Verification items for the finished model (mm, model axes). A direction names the side the tool comes from. Round coordinates to 2 decimals unless told otherwise and drop trailing zeros. Loops run counter-clockwise (first coordinate to the right, second up) from the corner with the lowest first, then second, coordinate; pieces in that order, holes last. Notation, with made-up numbers: M -24.75,10.25 L 33.25,10.25 A24 cw 33.25,37.25 Z; hole C 8,-25 d1. An arc over 180 degrees is marked long. One line per item, written item: value.
Autodesk Inventor part; units mm, degrees
ref_plane "YZ Plane" through (0, 0, 0) normal (1, 0, 0) x (0, 1, 0)
ref_plane "XZ Plane" through (0, 0, 0) normal (0, 1, 0) x (-1, 0, 0)
ref_plane "XY Plane" through (0, 0, 0) normal (0, 0, 1) x (1, 0, 0)
sketch "Sketch1" plane through (0, 0, 0) normal (0, 0, 1) x (1, 0, 0)
  circle A0 centre (0, 0) radius 38.1
  circle A1 centre (0, 0) radius 19.05
  dimension "d0" = 76.2
  dimension "d1" = 38.1
extrude "Extrusion1" add sketch "Sketch1" along normal blind 5.08
sketch "Sketch2" plane through (0, 0, 0) normal (0, 0, -1) x (-1, 0, 0)
  circle A0 centre (0, 0) radius 46.5667
  circle A1 centre (0, 0) radius 38.1
  dimension "d8" = 8.4667
extrude "Extrusion2" add sketch "Sketch2" against normal blind 20.2142
sketch "Sketch3" plane through (0, 0, 20.2142) normal (0, 0, 1) x (1, 0, 0)
  circle A0 centre (0, 0) radius 46.5667 construction
  arc A1 (23.2833, 40.3279) -> (0, 46.5667) centre (0, 0) ccw
  line L0 (0, 0) -> (23.2833, 40.3279) construction
  line L1 (0, 0) -> (0, 46.5667) construction
  circle A2 centre (0, 0) radius 38.1
  circle A3 centre (0, 0) radius 46.5667
  circle A4 centre (0, 0) radius 38.1
  line L2 (0, 38.1) -> (0, 46.5667)
  line L3 (19.05, 32.9956) -> (23.2833, 40.3279)
  arc A5 (19.05, 32.9956) -> (0, 38.1) centre (0, 0) ccw
  dimension "d9" = 30
extrude "Extrusion3" cut sketch "Sketch3" against normal blind 8.4667 contours L3 A2 L2 A1
pattern_circular "Circular Pattern1" count 6 over 360 about axis through (0, 0, 0) along (0, 0, 1) of "Extrusion3"
sketch "Sketch4" plane through (0, 0, 20.2142) normal (0, 0, 1) x (1, 0, 0)
  line L0 (-40.8909, 10.9567) -> (-10.9567, 40.8909)
  line L1 (-10.9567, 40.8909) -> (29.9342, 29.9342)
  line L2 (29.9342, 29.9342) -> (40.8909, -10.9567)
  line L3 (40.8909, -10.9567) -> (10.9567, -40.8909)
  line L4 (10.9567, -40.8909) -> (-29.9342, -29.9342)
  line L5 (-29.9342, -29.9342) -> (-40.8909, 10.9567)
  line L6 (-23.2833, 40.3279) -> (-19.05, 32.9956)
  arc A0 (0, 38.1) -> (-19.05, 32.9956) centre (0, 0) ccw
  line L7 (0, 38.1) -> (0, 46.5667)
  arc A1 (0, 46.5667) -> (-23.2833, 40.3279) centre (0, 0) ccw
  arc A2 (0, 38.1) -> (-19.05, 32.9956) centre (0, 0) ccw
  line L8 (-9.861, 36.8018) -> (-12.0523, 44.9799)
  arc A3 (0, 46.5667) -> (-23.2833, 40.3279) centre (0, 0) ccw
hole "Hole1" at (-10.9567, 40.8909, 20.2142) at (29.9342, 29.9342, 20.2142) at (-40.8909, 10.9567, 20.2142) at (-29.9342, -29.9342, 20.2142) at (10.9567, -40.8909, 20.2142) at (40.8909, -10.9567, 20.2142) direction (0, 0, -1) diameter 6 end through all
properties part number "Stator"
(1) Tool access check on faces 1 (the face through (0, -42, 16)), 2 (the face through (0, 42, 16)), 3 (the face through (40, 10, 11.748)). Record the directions out of +Z, -Z, +X, -X, +Y, -Y that give a thin tool (end or side, any length) a straight path to the whole face; none if there is none.
Completed:
face 1: +Z, -Y
face 2: +Z, +Y
face 3: +Z, +X
(2) Sectioned sample at D-D on z = 2.75. Enter the section's corners in (x, y), and give its area (3 significant figures).
Completed:
outline: C 0,0 d93.13; hole C -40.89,10.96 d6; hole C -29.93,-29.93 d6; hole C 0,0 d38.1; hole C -10.96,40.89 d6; hole C 10.96,-40.89 d6; hole C 29.93,29.93 d6; hole C 40.89,-10.96 d6
area: 5,500 mm^2
(3) Sectioned sample at A-A on z = 16.75. Count the separate pieces of the cut face and the enclosed holes in it, and give its area (3 significant figures).
Completed:
separate pieces: 6
enclosed holes: 6
area: 956 mm^2
(4) Depth check by flat-ended pin: pin 1 Ø1 at (y, z) = (-14.5, 5.5) entering from -X; pin 2 Ø2 at (y, z) = (-13, 10) entering from +X; pin 3 Ø11 at (x, y) = (-13.5, -40.5) entering from +Z. Enter the tip coordinate at first touch or a pass-through.
Completed:
pin 1: stops at x = -44.41
pin 2: stops at x = 44.99
pin 3: stops at z = 11.75
(5) Thickness scan on L1, parallel to Y at x = 29.5, z = 11; L2, parallel to X at y = -31.5, z = 9.25; L3, parallel to Z at x = -19, y = -26. Record the ranges inside material, lowest first. Write a range as from..to.
Completed:
L1: y = -36.03..-24.11, 24.11..26.97, 32.9..36.03
L2: x = -34.3..-32.49, -27.38..-21.43, 21.43..34.3
L3: z = 0..5.08
(6) Sectioned sample at C-C on x = -16. Enter the section's corners in (y, z).
Completed:
outline: M -43.73,0 L -10.34,0 L -10.34,5.08 L -34.58,5.08 L -34.58,11.75 L -43.73,11.75 Z; M 10.34,0 L 43.73,0 L 43.73,20.21 L 34.58,20.21 L 34.58,5.08 L 10.34,5.08 Z
(7) Mould release check, pull along Y, two halves, no side actions. Record for faces 4 (the face through (21.137, 36.61, 16.04)), 5 (the face through (-40, -10, 11.748)), 6 (the face through (-11, -40, 11.748)): +Y half, -Y half, draft (parallel to the pull), parting line (faces both ways), or undercut.
Completed:
face 4: +Y half
face 5: undercut
face 6: draft
(8) Sectioned sample at B-B on y = 2.5. Enter the section's corners in (x, z).
Completed:
outline: M -46.5,0 L -18.89,0 L -18.89,5.08 L -38.02,5.08 L -38.02,20.21 L -46.5,20.21 Z; M 18.89,0 L 46.5,0 L 46.5,11.75 L 38.02,11.75 L 38.02,5.08 L 18.89,5.08 Z
